```python
from build123d import *

# Parameters (mm, degrees)
SKETCH1_R           = 2.5
BOSS_EXTRUDE1_DEPTH = 4
FILLET1_R           = 0.5
FILLET4_R           = 0.5
FILLET5_R           = 0.5


with BuildPart() as part:
    # Sketch1 → Boss-Extrude1 (new body)
    with BuildSketch(Plane(origin=(0, 0, 0), x_dir=(1, 0, 0), z_dir=(0, 1, 0))):
        Polygon((-4.618802154, 0), (-2.309401077, -4), (2.309401077, -4), (4.618802154, 0), (2.309401077, 4), (-2.309401077, 4), align=None)
        Circle(SKETCH1_R, mode=Mode.SUBTRACT)
    extrude(amount=BOSS_EXTRUDE1_DEPTH)

    # Fillet1
    fillet1_edges = [part.edges().sort_by_distance(p)[0] for p in [
        (0, 4, -4),
        (-3.464101615, 4, -2),
        (-3.464101615, 4, 2),
        (0, 4, 4),
        (3.464101615, 4, 2),
        (3.464101615, 4, -2),
    ]]
    fillet(fillet1_edges, radius=FILLET1_R)

    # Fillet4
    fillet4_edges = [part.edges().sort_by_distance(p)[0] for p in [
        (-2.5, 0, 0),
        (0, 0, 4),
        (-3.464101615, 0, 2),
        (-3.464101615, 0, -2),
        (0, 0, -4),
        (3.464101615, 0, -2),
        (3.464101615, 0, 2),
    ]]
    fillet(fillet4_edges, radius=FILLET4_R)

    # Fillet5
    fillet5_edges = [part.edges().sort_by_distance(p)[0] for p in [
        (-2.5, 4, 0),
    ]]
    fillet(fillet5_edges, radius=FILLET5_R)


solid = part.part
```
Here's how the part is built. I have some questions about the finished solid (model axes, mm). Round coordinates to 2 decimals unless told otherwise and drop trailing zeros. Write each loop counter-clockwise with the first axis right and the second up, starting at its lowest first coordinate (ties: lowest second). Pieces come first, ordered by that corner, then holes. Notation, with made-up numbers: M -28,36.5 L -4,36.5 A11 cw -4,50.5 Z; hole C 18.5,29.25 d4. An arc over 180 degrees is marked long. Answer as CSV lines item,"result". Start each with the question number.
1. Suppose I cut it at B-B on y = 2.6. Write out the boundary of the cut face in (x, z), then the cut area to 3 significant figures.
2. Suppose I cut it at A-A on x = 0. Write out the boundary of the cut face in (y, z), then the cut area to 3 significant figures.
3. Thinking about a two-plate mould opening in Z: for faces 1 (the flat face through (3.48, 1.98, -1.97)), 2 (the cylindrical face through (3.35, 0.143, 1.897)), 3 (the flat face through (-1, 0, -3)), 4 (the cylindrical face through (-0.54, 1.98, 2.44)), which applies, released by +Z, released by -Z, zero draft, split by the parting line, or undercut?
4. I need wall thicknesses on probe 1 along Z at (x, y) = (0, 2.4); probe 2 along X at (y, z) = (2.05, 2.25); probe 3 along X at (y, z) = (1.7, -0.5). Which ranges of each line are inside material? Lowest first, please.
Check result:
1,outline,"M -4.62,0 L -2.31,-4 L 2.31,-4 L 4.62,0 L 2.31,4 L -2.31,4 Z; hole C 0,0 d5"
1,area,"35.8 mm2"
2,outline,"M 0,-3.5 A0.5 ccw 0.5,-4 L 3.5,-4 A0.5 ccw 4,-3.5 L 4,-3 A0.5 ccw 3.5,-2.5 L 0.5,-2.5 A0.5 ccw 0,-3 Z; M 0,3 A0.5 ccw 0.5,2.5 L 3.5,2.5 A0.5 ccw 4,3 L 4,3.5 A0.5 ccw 3.5,4 L 0.5,4 A0.5 ccw 0,3.5 Z"
2,area,"11.6 mm2"
3,face 1,"released by -Z"
3,face 2,"released by +Z"
3,face 3,"zero draft"
3,face 4,"undercut"
4,probe 1,"z = -4 to -2.5, 2.5 to 4"
4,probe 2,"x = -3.32 to -1.09, 1.09 to 3.32"
4,probe 3,"x = -4.33 to -2.45, 2.45 to 4.33"
